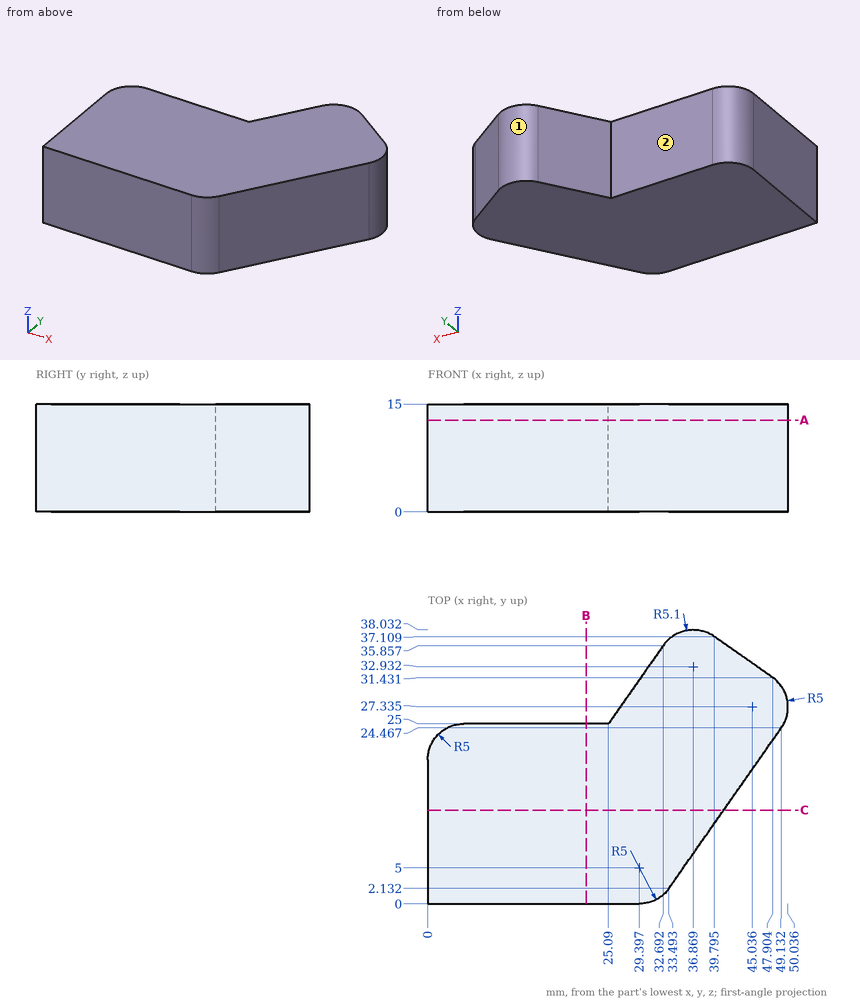
Geometry check sheet. Reference: drawing and pictorial views, mm from the part's lowest x, y, z. A direction names the side the tool comes from. Give positions to 0.01 mm unless a question says otherwise; leave off trailing zeros. Loops run counter-clockwise (first coordinate to the right, second up) from the corner with the lowest first, then second, coordinate; pieces in that order, holes last.
1. Go/stop test with flat-tipped pins: pin 1 Ø5 at (x, z) = (44.5, 8) entering from +Y (1 decimal); pin 2 Ø8 at (y, z) = (12, 13.5) entering from +X; pin 3 Ø5 at (x, z) = (12, 9) entering from +Y. Record where each tip stops, or that it passes through.
2. Section check C-C, the plane y = 13. Enter the section's corners in (x, z).
3. Set-up check for the marked faces 1 and 2: record each of +Z, -Z, +X, -X, +Y, -Y from which the full face is reachable in a straight line by a thin tool's end or side.
4. Section check A-A, the plane z = 12.75. Enter the section's corners in (x, y) (1 decimal), then the cut area to 3 significant figures.
5. Thickness scan on line 1 (Y direction, x = 23, z = 10.75); line 2 (Y direction, x = 42.5, z = 8.75) (1 decimal); line 3 (X direction, y = 20.5, z = 8) (1 decimal). Record the ranges inside material, lowest first.
6. Section check B-B, the plane x = 22. Enter the section's corners in (y, z), then the cut area to 3 significant figures.
Geometry says:
1. pin 1: stops at y = 35.6
1. pin 2: stops at x = 43.2
1. pin 3: stops at y = 25
2. outline: (0, 0) - (41.1, 0) - (41.1, 15) - (0, 15) - close
3. face 1: +Z, -Z, +Y
3. face 2: +Z, -Z, -X, +Y
4. outline: (0, 0) - (29.4, 0) arc R5 ccw to (33.5, 2.1) - (49.1, 24.5) arc R5 ccw to (47.9, 31.4) - (39.8, 37.1) arc R5.1 ccw to (32.7, 35.9) - (25.1, 25) - (5, 25) arc R5 ccw to (0, 20) - close
4. area: 1,230 mm2
5. line 1: y = 0 to 25
5. line 2: y = 15 to 35.2
5. line 3: x = 0 to 46.4
6. outline: (0, 0) - (25, 0) - (25, 15) - (0, 15) - close
6. area: 375 mm2
